```python
from build123d import *

# Parameters (mm, degrees)
SKETCH1_R           = 4.7625
BOSS_EXTRUDE1_DEPTH = 3.175
SKETCH2_R           = 29.21
SKETCH2_R_2         = 22.86
CUT_EXTRUDE1_DEPTH  = 7.62
SKETCH5_R           = 38.1
SKETCH5_R_2         = 25.4
CUT_EXTRUDE5_DEPTH  = 12.7


with BuildPart() as part:
    # Sketch1 → Boss-Extrude1 (new body)
    with BuildSketch(Plane.XY):
        Polygon((0, 0), (-40.591135768, 23.435303163), (-65.991135768, -20.55878735), (0, -58.65878735), (64.135, -58.65878735), (64.135, -51.03878735), (70.612, -51.03878735), (70.612, -58.65878735), (95.758, -58.65878735), (95.758, -51.03878735), (102.235, -51.03878735), (102.235, -58.65878735), (166.37, -58.65878735), (166.37, -101.6), (234.95, -101.6), (234.95, 0), align=None)
        with Locations((-20.295567884, -17.611742094)):
            Circle(SKETCH1_R, mode=Mode.SUBTRACT)
        with Locations((-53.291135768, -17.611742094)):
            Circle(SKETCH1_R, mode=Mode.SUBTRACT)
        with Locations((-36.793351826, 10.963257906)):
            Circle(SKETCH1_R, mode=Mode.SUBTRACT)
        with Locations((7.62, -51.03878735)):
            Circle(SKETCH1_R, mode=Mode.SUBTRACT)
        with Locations((7.62, -7.62)):
            Circle(SKETCH1_R, mode=Mode.SUBTRACT)
        with Locations((48.895, -7.62)):
            Circle(SKETCH1_R, mode=Mode.SUBTRACT)
        with Locations((117.475, -7.62)):
            Circle(SKETCH1_R, mode=Mode.SUBTRACT)
        with Locations((147.32, -7.62)):
            Circle(SKETCH1_R, mode=Mode.SUBTRACT)
        with Locations((117.475, -51.03878735)):
            Circle(SKETCH1_R, mode=Mode.SUBTRACT)
        with Locations((48.895, -51.03878735)):
            Circle(SKETCH1_R, mode=Mode.SUBTRACT)
        with Locations((147.32, -51.03878735)):
            Circle(SKETCH1_R, mode=Mode.SUBTRACT)
        with Locations((176.53, -20.32)):
            Circle(SKETCH1_R, mode=Mode.SUBTRACT)
        with Locations((201.93, -20.32)):
            Circle(SKETCH1_R, mode=Mode.SUBTRACT)
        with Locations((227.33, -7.62)):
            Circle(SKETCH1_R, mode=Mode.SUBTRACT)
        with Locations((227.33, -93.98)):
            Circle(SKETCH1_R, mode=Mode.SUBTRACT)
        with Locations((176.53, -93.98)):
            Circle(SKETCH1_R, mode=Mode.SUBTRACT)
        with Locations((227.33, -51.03878735)):
            Circle(SKETCH1_R, mode=Mode.SUBTRACT)
        with Locations((176.53, -51.03878735)):
            Circle(SKETCH1_R, mode=Mode.SUBTRACT)
    extrude(amount=BOSS_EXTRUDE1_DEPTH)

    # Sketch2 → Cut-Extrude1 (cut)
    with BuildSketch(Plane.XZ.offset(58.65878735)):
        with Locations((83.185, 22.225)):
            Circle(SKETCH2_R)
        with Locations((83.185, 22.225)):
            Circle(SKETCH2_R_2, mode=Mode.SUBTRACT)
    extrude(amount=-CUT_EXTRUDE1_DEPTH, mode=Mode.SUBTRACT)

    # Sketch5 → Cut-Extrude5 (cut)
    with BuildSketch(Plane(origin=(0, 0, 0), x_dir=(1, 0, 0), z_dir=(0, 1, 0))):
        with Locations((185.42, -22.225)):
            Circle(SKETCH5_R)
        with Locations((83.312, -22.225)):
            Circle(SKETCH5_R_2)
    extrude(amount=-CUT_EXTRUDE5_DEPTH, mode=Mode.SUBTRACT)


solid = part.part
```
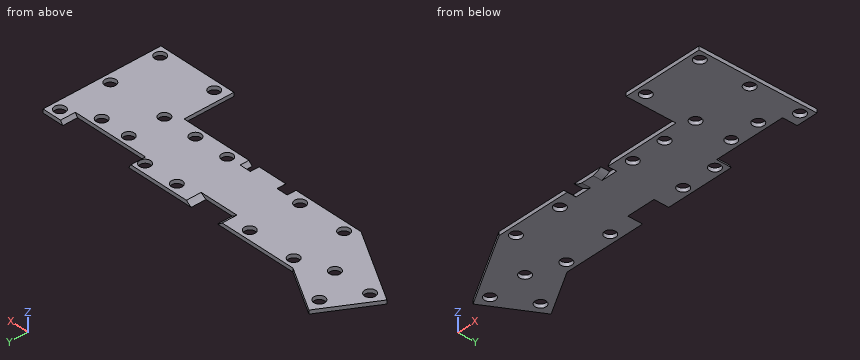
Build history of the part. All positions in model axes, mm. Give positions to 0.01 mm unless a question says otherwise; leave off trailing zeros. Loops run counter-clockwise (first coordinate to the right, second up) from the corner with the lowest first, then second, coordinate; pieces in that order, holes last.
Item 1: Slice it at A-A, the plane x = 201.93. List the corners of the cut face in (y, z) (1 decimal), and give its area (3 significant figures).
Answers follow:
outline: (-101.6, 0) - (-25.1, 0) - (-25.1, 3.2) - (-101.6, 3.2) - close; (-15.6, 0) - (-12.7, 0) - (-12.7, 3.2) - (-15.6, 3.2) - close
area: 252 mm2
Item 2: Slice it at B-B, the plane x = 147.32. List the corners of the cut face in (y, z) (1 decimal), and give its area (3 significant figures).
Answers follow:
outline: (-58.7, 0) - (-55.8, 0) - (-55.8, 3.2) - (-58.7, 3.2) - close; (-46.3, 0) - (-12.4, 0) - (-12.4, 3.2) - (-46.3, 3.2) - close; (-2.9, 0) - (0, 0) - (0, 3.2) - (-2.9, 3.2) - close
area: 126 mm2
Item 3: Slice it at C-C, the plane y = -85.5. List the corners of the cut face in (x, z) (3 decimals).
Answers follow:
outline: (166.37, 0) - (234.95, 0) - (234.95, 3.175) - (166.37, 3.175) - close
Item 4: Slice it at D-D, the plane x = 117. List the corners of the cut face in (y, z) (3 decimals).
Answers follow:
outline: (-58.659, 0) - (-55.778, 0) - (-55.778, 3.175) - (-58.659, 3.175) - close; (-46.3, 0) - (-12.359, 0) - (-12.359, 3.175) - (-46.3, 3.175) - close; (-2.881, 0) - (0, 0) - (0, 3.175) - (-2.881, 3.175) - close
Item 5: Drill centre lines: line 1 (Y direction, x = 176.53, z = 0.85); line 2 (X direction, y = -24, z = 1); line 3 (X direction, y = -20, z = 0.75). Where is each one in solid material? Low to high.
Answers follow:
line 1: y = -101.6 to -98.74, -89.22 to -55.8, -46.28 to -25.08, -15.56 to -12.7
line 2: x = -60.03 to 173.51, 179.55 to 198.91, 204.95 to 234.95
line 3: x = -65.67 to -57.41, -49.17 to -24.42, -16.18 to 171.78, 181.28 to 197.18, 206.68 to 234.95
Item 6: Flat gauge pins, fed straight in: pin 1 (1 mm diameter, centred on x = 33, z = 2, fed in from -Y); pin 2 (1.6 mm diameter, centred on x = 118, z = 2, fed in from +Y). Where does each tip first touch, or does it go through?
Answers follow:
pin 1: stops at y = -58.66
pin 2: stops at y = 0
